Part model, mm, in its own coordinate system. Give positions to 0.01 mm unless a question says otherwise; leave off trailing zeros. Order: outer loops, then holes, each group sorted by start corner. A loop starts at its lowest first (then second) coordinate and runs counter-clockwise, first axis right, second up. Notation, with made-up numbers: (70.5, 9) -> (112.5, 9) arc R12 cw to (112.5, 13) -> close; hole circle Ø1 at (66, -5). An arc over 180 degrees is marked (long way). Write item = value, one per line. Start each with the question number.
(1) Saw through at B-B, the plane z = 4.75. List the corners of the cut face in (x, y), then the cut area to 3 significant figures.
(2) Probe line 1 along X through (y, z) = (-2.05, 4.75); line 2 along X through (y, z) = (-1.6, 9.25); line 3 along Y through (x, z) = (23.5, 3.25). List the from-to ranges inside material, lowest first. Write a range as from..to.
(3) Saw through at C-C, the plane x = 23. List the corners of the cut face in (y, z).
(4) Two-plate mould, pull along X, no slides. Class faces 1 (the flat face through (14.637, 0, 5)), 2 (the cylindrical face through (22.7, -1, 5.1)), 3 (the flat face through (20, 2.5, 5)): pulls with the +X half, pulls with the -X half, needs draft (parallel to the pull), parting line crosses it, or undercut.
(5) Saw through at A-A, the plane y = -1.3. List the corners of the cut face in (x, z).
from build123d import *

# Parameters (mm, degrees)
F0_W     = 11
F0_H     = 5
F1_DEPTH = 10
F3_DEPTH = 10.001


with BuildPart() as f1:
    # F0 (on Top) → F1 (new body)
    with BuildSketch(Plane.XY):
        with Locations((20.1367214707, 0)):
            Rectangle(F0_W, F0_H)
    extrude(amount=F1_DEPTH)

    # F2 (on face) → F3 (cut, through all)
    with BuildSketch(Plane.XY.offset(10)):
        with BuildLine():
            Line((21.1367214707, -2.5), (24.1367214707, -2.5))
            ThreePointArc((24.1367214707, -2.5), (22.6367214707, -1), (21.1367214707, -2.5))
        make_face()
    extrude(amount=-F3_DEPTH, mode=Mode.SUBTRACT)


solid = f1.part
Results list:
q1.outline = (14.64, -2.5) -> (21.14, -2.5) arc R1.5 cw to (24.14, -2.5) -> (25.64, -2.5) -> (25.64, 2.5) -> (14.64, 2.5) -> close
q1.area = 51.5 mm^2
q2.line_1 = 14.64..21.21, 24.07..25.64
q2.line_2 = 14.64..21.44, 23.84..25.64
q2.line_3 = -1.27..2.5
q3.outline = (-1.04, 0) -> (2.5, 0) -> (2.5, 10) -> (-1.04, 10) -> close
q4.face_1 = pulls with the -X half
q4.face_2 = undercut
q4.face_3 = needs draft
q5.outline = (14.64, 0) -> (21.74, 0) -> (21.74, 10) -> (14.64, 10) -> close; (23.54, 0) -> (25.64, 0) -> (25.64, 10) -> (23.54, 10) -> close
